For this review, take the finished solid that the model builds, in its own axes (mm). A direction names the side the tool comes from. Round coordinates to 2 decimals unless told otherwise and drop trailing zeros. Write each loop counter-clockwise with the first axis right and the second up, starting at its lowest first coordinate (ties: lowest second). Pieces come first, ordered by that corner, then holes. Notation, with made-up numbers: (83, -1.75) -> (90, -1.75) arc R23 ccw to (90, 37.25) -> close; hole circle Ø1 at (83.5, -33.75). An arc over 180 degrees is marked (long way). Write item = value, one per line. Start each with the question number.
Autodesk Inventor part; units mm, degrees
ref_plane "Start Plane" through (0, 0, 0) normal (0, 0, 1) x (1, 0, 0)
ref_plane "End Plane" through (0, 0, 1000) normal (0, 0, 1) x (1, 0, 0)
ref_plane "YZ Plane" through (0, 0, 0) normal (1, 0, 0) x (0, 1, 0)
ref_plane "Start Plane" through (0, 0, 0) normal (0, 0, 1) x (1, 0, 0)
ref_plane "End Plane" through (0, 0, 1000) normal (0, 0, 1) x (1, 0, 0)
sketch "Sketch" plane through (0, 0, 0) normal (0, 0, 1) x (1, 0, 0)
  line L0 (28.702, 0) -> (0, 0)
  line L1 (0, 0) -> (0, 28.702)
  line L2 (0, 28.702) -> (1.905, 28.702)
  line L3 (3.175, 27.432) -> (3.175, 5.461)
  line L4 (5.461, 3.175) -> (27.432, 3.175)
  line L5 (28.702, 1.905) -> (28.702, 0)
  line L6 (0, -11.0414) -> (0, 31.5385) construction
  line L7 (-11.0414, 0) -> (31.5385, 0) construction
  arc A0 (3.175, 5.461) -> (5.461, 3.175) centre (5.461, 5.461) ccw
  arc A1 (3.175, 27.432) -> (1.905, 28.702) centre (1.905, 27.432) ccw
  arc A2 (28.702, 1.905) -> (27.432, 3.175) centre (27.432, 1.905) ccw
  line L8 (0, 40.0545) -> (0, -19.5574) construction
  line L9 (-19.5574, 0) -> (40.0545, 0) construction
  point P0 (3.175, 28.702)
  point P1 (3.175, 3.175)
  point P2 (28.702, 3.175)
  dimension "d0" = 28.702
  dimension "d1" = 28.702
  dimension "d2" = 3.175
  dimension "d3" = 3.175
  dimension "d10" = 0
  dimension "d11" = 0
  dimension "d14" = 2.286
  dimension "d15" = 1.27
extrude "Body" add sketch "Sketch" along normal up to surface (1000 mm away) from surface at 0
sketch "Sketch3" plane through (0, 0, 0) normal (0, 0, 1) x (1, 0, 0)
  line L0 (0, 0) -> (10, 0)
ref_plane "Work Plane3" through (0, 0, 0) normal (0, -1, 0) x (1, 0, 0)
sketch "Sketch4" plane through (0, 0, 0) normal (0, -1, 0) x (1, 0, 0)
  line L0 (-2, 0) -> (12, 0)
  line L1 (-2, 1000) -> (12, 1000)
  dimension "d17" = 1000
equation "\"d0\" = G_H"
equation "\"d1\" = G_H"
equation "\"d2\" = G_T"
equation "\"d3\" = G_T"
equation "\"d14\" = G_IR"
equation "\"d15\" = G_ER"
equation "\"d4\" = G_L"
equation "\"G_H\" = 28.702"
equation "\"G_T\" = 3.175"
equation "\"G_ER\" = 1.27"
equation "\"G_IR\" = 2.286"
equation "\"G_L\" = d17"
equation "\"ex\" = 0"
equation "\"G_OFFSET_START\" = 0"
equation "\"G_OFFSET_END\" = 0"
properties part number "AISC - L 1.13 x 1.13 x 1/8 - 39.37" material "Steel, Mild"
1. Consider section A-A, the plane z = 640. Give the boundary of the cut face in (x, y) (3 decimals), then the cut area to 3 significant figures.
2. Consider section B-B, the plane x = 19. Give the boundary of the cut face in (y, z) (3 decimals).
3. Machinability: for faces 1 (the flat face through (16, 3.175, 493)), 2 (the flat face through (15, 0, 493)), which of the approach directions +Z, -Z, +X, -X, +Y, -Y give a long, thin tool a straight path to every point of the face, cutting with its end or side? Answer none if there is none.
4. Draft analysis for pull direction Z (two halves, no side actions). For faces 3 (the flat face through (3, 8, 1000)), 4 (the flat face through (3.175, 17, 493)), 5 (the flat face through (3, 8, 0)), state which applies: +Z half, -Z half, draft (parallel to the pull), parting line (faces both ways), or undercut.
5. Wall thickness on L1, parallel to X at y = 27.25, z = 516 (3 decimals); L2, parallel to X at y = 2.5, z = 246.5: over which ranges is each line inside the solid? List them lowest first. Write a range as from..to.
6. Clearance check with flat-ended pins moving along their axes: pin 1 Ø6.5 at (y, z) = (20.5, 667.5) entering from +X (3 decimals); pin 2 Ø4 at (x, z) = (24.5, 525.5) entering from +Y (3 decimals); pin 3 Ø10 at (x, z) = (8, 105) entering from +Y. State where each tip first meets the part, or that it passes through.
Outcome:
q1.outline = (0, 0) -> (28.702, 0) -> (28.702, 1.905) arc R1.27 ccw to (27.432, 3.175) -> (5.461, 3.175) arc R2.286 cw to (3.175, 5.461) -> (3.175, 27.432) arc R1.27 ccw to (1.905, 28.702) -> (0, 28.702) -> close
q1.area = 173 mm2
q2.outline = (0, 0) -> (3.175, 0) -> (3.175, 1000) -> (0, 1000) -> close
q3.face_1 = +Z, -Z, +X, +Y
q3.face_2 = +Z, -Z, +X, -X, -Y
q4.face_3 = +Z half
q4.face_4 = draft
q4.face_5 = -Z half
q5.L1 = 0..3.175
q5.L2 = 0..28.55
q6.pin_1 = 3.175
q6.pin_2 = 3.175
q6.pin_3 = 28.08
